Check sheet for the drawn part. Datum: minimum x, y, z corner. Units: mm. Coordinates: 2 decimals unless noted, no trailing zeros. Loops run counter-clockwise (first coordinate to the right, second up) from the corner with the lowest first, then second, coordinate; pieces in that order, holes last.
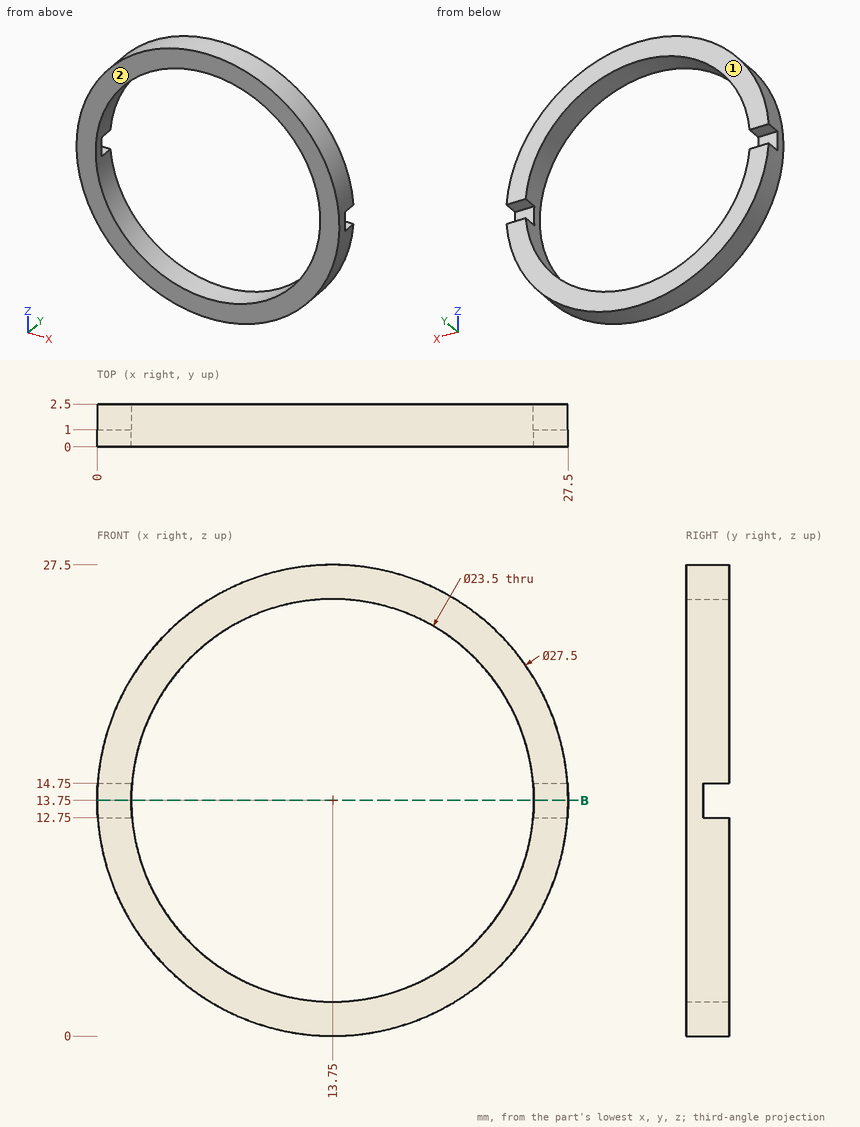
(1) Gauge pin test, flat ends, axial feed: pin 1 Ø1.5 at (y, z) = (1.5, 7.5) entering from +X; pin 2 Ø1 at (y, z) = (1.5, 21) entering from -X; pin 3 Ø1.2 at (x, y) = (1, 1.5) entering from +Z. Record the tip position at first contact, or that the pin passes through.
Findings:
pin 1: stops at x = 26.35
pin 2: stops at x = 1.77
pin 3: stops at z = 20.19
(2) Draft check along Y on the marked faces 1 and 2. Enter one of: +Y half, -Y half, draft (parallel to the pull), parting line (faces both ways), or undercut.
Findings:
face 1: +Y half
face 2: -Y half
(3) Scan lines: L1, parallel to X at y = 0.85, z = 13.75; L2, parallel to Z at x = 11, y = 2.05; L3, parallel to Z at x = 18, y = 0.7. Record each from-to range of solid material in increasing order.
Findings:
L1: x = 0 to 2, 25.5 to 27.5
L2: z = 0.28 to 2.33, 25.17 to 27.22
L3: z = 0.67 to 2.8, 24.7 to 26.83
(4) Sectioned sample at B-B on z = 13.75. Record the cut outline in (x, y).
Findings:
outline: (0, 0) - (2, 0) - (2, 1) - (0, 1) - close; (25.5, 0) - (27.5, 0) - (27.5, 1) - (25.5, 1) - close
